Geometry: final body of the model. Coordinates: model frame, mm. Face numbers are marked on the shaded views. A direction names the side the tool comes from. Round coordinates to 2 decimals unless told otherwise and drop trailing zeros. Loops run counter-clockwise (first coordinate to the right, second up) from the corner with the lowest first, then second, coordinate; pieces in that order, holes last. Notation, with made-up numbers: (84, -8.5) - (121, -8.5) arc R25 ccw to (121, 27.5) - close; hole circle Ø10 at (-2.5, 24.5). An arc over 180 degrees is marked (long way). Answer as a JSON object with one key per item and string values. Group by question number.
Item 1: Section B-B (x = -39.5). Return the cut outline in (y, z).
Item 2: First-contact query: pin 1 (5 mm diameter, centred on y = 28, z = 11.5, fed in from -X); pin 2 (4 mm diameter, centred on x = -31, z = 34, fed in from +Y); pin 3 (4 mm diameter, centred on x = -21.5, z = 7.5, fed in from +Y). Flat tips, straight axial feed; report the tip coordinate or a pass-through.
Item 3: Section A-A (y = 19). Return the cut outline in (x, z), plus the area to 3 significant figures.
Item 4: Draft query along Z for the marked faces 1, 2 and 3. Return one class per face: released by +Z, released by -Z, zero draft, split by the parting line, or undercut.
Item 5: Section C-C (x = -50.5). Return the cut outline in (y, z).
Item 6: Reachability of the marked faces 4, 5 and 6 from +Z, -Z, +X, -X, +Y, -Y: full face, straight path, thin tool, end or side. Return the list, or none.
Item 7: Line query: line 1 (Z direction, x = -15.5, y = 15.5); line 2 (X direction, y = 7.5, z = 28); line 3 (X direction, y = 20.5, z = 29). Output: solid intervals per line, ascending.
```python
from build123d import *

# Parameters (mm, degrees)
EXTRUDE_1_DEPTH     = 2
SKETCH_2_W          = 6
SKETCH_2_H          = 35
EXTRUDE_2_DEPTH     = 60
FILLET_1_R          = 17.5
SKETCH_3_R          = 16
CUT_EXTRUDE_1_DEPTH = 5
CHAMFER_1_SIZE      = 1.640243073
CHAMFER_1_SIZE_2    = 0.8
SKETCH_4_R          = 15
CUT_EXTRUDE_2_DEPTH = 105.385422037
SKETCH_5_W          = 25
SKETCH_5_H          = 10.5
EXTRUDE_3_DEPTH     = 7.3
EXTRUDE_4_DEPTH     = 2
FILLET_2_R          = 1
EXTRUDE_5_DEPTH     = 5
SKETCH_9_R          = 1.15
CUT_EXTRUDE_3_DEPTH = 101.277297201
SKETCH_10_R         = 2
CUT_EXTRUDE_4_DEPTH = 10
FILLET_3_R          = 0.5
SKETCH_12_W         = 56.21
SKETCH_12_H         = 29.03
CUT_EXTRUDE_5_DEPTH = 113.159332301


# Some blends are built 0.0001 mm under size
with BuildPart() as part:
    # 스케치1 → 보스-돌출1 (new body)
    with BuildSketch(Plane(origin=(0, 0, 0), x_dir=(1, 0, 0), z_dir=(0, 1, 0))):
        with BuildLine():
            Line((-11.24267666, -2.527135016), (-67.45267666, -2.527135016))
            ThreePointArc((-67.45267666, -2.527135016), (-50.72671765, -44.531450868), (-11.24267666, -66.557135016))
            Line((-11.24267666, -66.557135016), (-11.24267666, -2.527135016))
        make_face()
    extrude(amount=EXTRUDE_1_DEPTH)

    # 스케치2 → 보스-돌출2 (add)
    with BuildSketch(Plane(origin=(0, 2, 0), x_dir=(1, 0, 0), z_dir=(0, 1, 0))):
        with Locations((-14.24267666, -20.027135016)):
            Rectangle(SKETCH_2_W, SKETCH_2_H)
    extrude(amount=EXTRUDE_2_DEPTH)

    # 필렛1
    fillet_1_edges = [part.edges().sort_by_distance(p)[0] for p in [
        (-14.24267666, 62, 2.527135016),
        (-14.24267666, 62, 37.527135016),
    ]]
    fillet(fillet_1_edges, radius=FILLET_1_R - 0.0001)  # a hair under: the kernel refuses the full size

    # 스케치3 → 컷-돌출1 (cut)
    with BuildSketch(Plane(origin=(-11.24267666, 0, 0), x_dir=(0, 0, -1), z_dir=(1, 0, 0))):
        with Locations((-20.027135016, 44.5)):
            Circle(SKETCH_3_R)
    extrude(amount=-CUT_EXTRUDE_1_DEPTH, mode=Mode.SUBTRACT)

    # 모따기1
    # the kernel refuses this chamfer: 1.640243073, 0.8 mm, written as the material it takes off along each edge
    with BuildSketch(Plane(origin=(-11.24267666, 44.5, 20.027135016), x_dir=(0, 0, -1), z_dir=(0, -1, 0))) as chamfer_1_piece_1:
        Polygon((16 + CHAMFER_1_SIZE, 0), (16, -CHAMFER_1_SIZE_2), (16, 0), align=None)
    revolve(axis=Axis((-11.24267666, 44.5, 20.027135016), (1, 0, 0)), mode=Mode.SUBTRACT)

    # 스케치4 → 컷-돌출2 (cut, through all)
    with BuildSketch(Plane(origin=(-16.24267666, 0, 0), x_dir=(0, 0, -1), z_dir=(1, 0, 0))):
        with Locations((-20.027135016, 44.5)):
            Circle(SKETCH_4_R)
    extrude(amount=-CUT_EXTRUDE_2_DEPTH, mode=Mode.SUBTRACT)

    # 스케치5 → 보스-돌출3 (add)
    with BuildSketch(Plane(origin=(0, 2, 0), x_dir=(1, 0, 0), z_dir=(0, 1, 0))):
        with Locations((-32.74267666, -7.777135016)):
            Rectangle(SKETCH_5_W, SKETCH_5_H)
        with Locations((-32.74267666, -32.277135016)):
            Rectangle(SKETCH_5_W, SKETCH_5_H)
    extrude(amount=EXTRUDE_3_DEPTH)

    # 스케치6 → 보스-돌출4 (add)
    with BuildSketch(Plane(origin=(0, 9.3, 0), x_dir=(1, 0, 0), z_dir=(0, 1, 0))):
        Polygon((-45.24267666, -32.527135016), (-25.24267666, -32.527135016), (-25.24267666, -27.027135016), (-20.24267666, -27.027135016), (-20.24267666, -37.527135016), (-45.24267666, -37.527135016), align=None)
        Polygon((-45.24267666, -2.527135016), (-20.24267666, -2.527135016), (-20.24267666, -13.027135016), (-25.24267666, -13.027135016), (-25.24267666, -7.527135016), (-45.24267666, -7.527135016), align=None)
    extrude(amount=EXTRUDE_4_DEPTH)

    # 필렛2
    fillet_2_edges = [part.edges().sort_by_distance(p)[0] for p in [
        (-45.24267666, 6.65, 2.527135016),
        (-45.24267666, 5.65, 13.027135016),
        (-45.24267666, 5.65, 27.027135016),
        (-45.24267666, 6.65, 37.527135016),
    ]]
    fillet(fillet_2_edges, radius=FILLET_2_R)

    # 스케치7 → 보스-돌출5 (add)
    with BuildSketch(Plane.ZY.offset(25.24267666)):
        with BuildLine():
            Line((2.527135016, 11.3), (13.027135016, 11.3))
            Line((13.027135016, 11.3), (13.027135016, 36.014718626))
            ThreePointArc((13.027135016, 36.014718626), (10.875170651, 38.397414624), (9.502877322, 41.3))
            Line((9.502877322, 41.3), (2.527135016, 41.3))
            Line((2.527135016, 41.3), (2.527135016, 11.3))
        make_face()
        with BuildLine():
            Line((37.527135016, 11.3), (27.027135016, 11.3))
            Line((27.027135016, 11.3), (27.027135016, 36.014718626))
            ThreePointArc((27.027135016, 36.014718626), (29.17909938, 38.397414624), (30.551392709, 41.3))
            Line((30.551392709, 41.3), (37.527135016, 41.3))
            Line((37.527135016, 41.3), (37.527135016, 11.3))
        make_face()
    extrude(amount=-EXTRUDE_5_DEPTH)

    # 스케치9 → 컷-돌출3 (cut, through all)
    with BuildSketch(Plane.ZY.offset(25.24267666)):
        with Locations((9.777135016, 35.8)):
            Circle(SKETCH_9_R)
        with Locations((9.777135016, 15.3)):
            Circle(SKETCH_9_R)
        with Locations((30.277135016, 15.3)):
            Circle(SKETCH_9_R)
        with Locations((30.277135016, 35.8)):
            Circle(SKETCH_9_R)
    extrude(amount=-CUT_EXTRUDE_3_DEPTH, mode=Mode.SUBTRACT)

    # 스케치10 → 컷-돌출4 (cut)
    with BuildSketch(Plane(origin=(-11.24267666, 0, 0), x_dir=(0, 0, -1), z_dir=(1, 0, 0))):
        with Locations((-30.277135016, 15.3)):
            Circle(SKETCH_10_R)
        with Locations((-9.777135016, 15.3)):
            Circle(SKETCH_10_R)
        with Locations((-9.777135016, 35.8)):
            Circle(SKETCH_10_R)
        with Locations((-30.277135016, 35.8)):
            Circle(SKETCH_10_R)
    extrude(amount=-CUT_EXTRUDE_4_DEPTH, mode=Mode.SUBTRACT)

    # 필렛3
    fillet_3_edges = [part.edges().sort_by_distance(p)[0] for p in [
        (-45.24267666, 10.3, 32.527135016),
        (-25.24267666, 22.657359313, 27.027135016),
        (-35.24267666, 9.3, 32.527135016),
        (-45.24267666, 9.3, 30.277135016),
        (-44.949783441, 9.3, 27.320028235),
        (-34.74267666, 9.3, 13.027135016),
        (-44.949783441, 9.3, 12.734241797),
        (-45.24267666, 9.3, 9.777135016),
        (-35.24267666, 9.3, 7.527135016),
        (-45.24267666, 10.3, 7.527135016),
        (-25.24267666, 22.657359313, 13.027135016),
        (-34.74267666, 9.3, 27.027135016),
    ]]
    fillet(fillet_3_edges, radius=FILLET_3_R)

    # 스케치12 → 컷-돌출5 (cut, through all)
    with BuildSketch(Plane(origin=(0, 2, 0), x_dir=(1, 0, 0), z_dir=(0, 1, 0))):
        with Locations((-39.34767666, -52.042135016)):
            Rectangle(SKETCH_12_W, SKETCH_12_H)
    extrude(amount=-CUT_EXTRUDE_5_DEPTH, mode=Mode.SUBTRACT)


solid = part.part
```
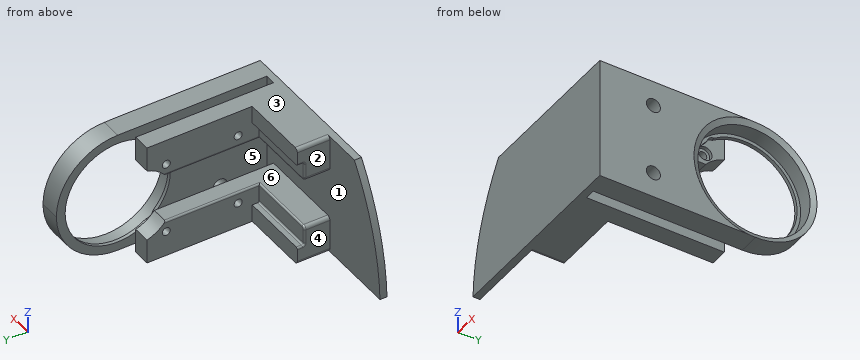
Values:
{
 "1": {"outline": "(0, 2.53) - (11.3, 2.53) - (11.3, 7.53) - (9.8, 7.53) arc R0.5 cw to (9.3, 8.03) - (9.3, 12.53) arc R0.5 ccw to (8.8, 13.03) - (2, 13.03) - (2, 27.03) - (8.8, 27.03) arc R0.5 ccw to (9.3, 27.53) - (9.3, 32.03) arc R0.5 cw to (9.8, 32.53) - (11.3, 32.53) - (11.3, 37.53) - (0, 37.53) - close"},
 "2": {"pin 1": "stops at x = -25.24", "pin 2": "stops at y = 11.3", "pin 3": "stops at y = 41.3"},
 "3": {"outline": "(-25.24, 2.53) - (-20.24, 2.53) - (-20.24, 13.03) - (-24.74, 13.03) arc R0.5 ccw to (-25.24, 12.53) - close; (-25.24, 27.53) arc R0.5 ccw to (-24.74, 27.03) - (-20.24, 27.03) - (-20.24, 37.53) - (-25.24, 37.53) - close; (-17.24, 2.53) - (-11.24, 2.53) - (-11.24, 37.53) - (-17.24, 37.53) - close", "area": "315 mm^2"},
 "4": {"face 1": "undercut", "face 2": "zero draft", "face 3": "released by +Z"},
 "5": {"outline": "(0, 2.53) - (2, 2.53) - (2, 37.53) - (0, 37.53) - close"},
 "6": {"face 4": "+Z, -Z, -X, +Y", "face 5": "+Z, -Z, +Y", "face 6": "-X, +Y"},
 "7": {"line 1": "z = 2.53 to 7.79, 11.77 to 28.29, 32.27 to 37.53", "line 2": "x = -45.24 to -20.24, -17.24 to -11.24", "line 3": "x = -25.24 to -20.24, -17.24 to -11.24"}
}
